Design review of the part built by this model. Coordinates are the model's own, in mm. A direction names the side the tool comes from. Coordinates: 2 decimals unless noted, no trailing zeros. Loops run counter-clockwise (first coordinate to the right, second up) from the corner with the lowest first, then second, coordinate; pieces in that order, holes last. Notation, with made-up numbers: (0, -20.5) - (51, -20.5) arc R11 cw to (51, -0.5) - close; hole circle Ø9 at (66, -3.75). An arc over 180 degrees is marked (long way). Answer in a Markdown table with one row per item. Add a question column.
(1) We need section C-C, the plane z = 31.5. Write out the cut boundary in (x, y), plus the area to 3 significant figures.
(2) Clearance check with flat-ended pins moving along their axes: pin 1 (4.5 mm diameter, centred on x = 10.5, y = -0.5, fed in from -Z); pin 2 (0.5 mm diameter, centred on x = -15.5, y = -4, fed in from -Z); pin 3 (12 mm diameter, centred on y = -0.5, z = 97, fed in from +X); pin 4 (1 mm diameter, centred on y = -4, z = 122, fed in from -X). State where each tip first meets the part, or that it passes through.
(3) To check wall thickness, follow L1, parallel to Z at x = 9, y = 8; L2, parallel to X at y = 0.5, z = 114; L3, parallel to Y at x = -0.5, z = 101. State the ranges of each line that lie inside material, in increasing order. Write a range as [from, to].
(4) For faces 1 (the face through (0, 14, 123)), 2 (the face through (-4.26, 0.03, 4.18)), 3 (the face through (-13.5, 0, 58)), 4 (the face through (11, 0, 8.477)), list the 3-axis set-ups (+Z, -Z, +X, -X, +Y, -Y) from which the entire face can be reached by the end or side of a thin tool; tool diameter is ignored.
(5) We need section B-B, the plane y = 5. Write out the cut boundary in (x, z), plus the area to 3 significant figures.
(6) The part is to be moulded in two halves that separate along X. For faces 5 (the face through (0, 2, 53)), 6 (the face through (0, -1, 108.5)), 7 (the face through (10.24, 0.03, 4.18)), say which applies: released by +X, released by -X, zero draft, split by the parting line, or undercut.
(7) We need section A-A, the plane x = 0.5. Write out the cut boundary in (y, z).
from build123d import *

# Parameters (mm, degrees)
ESQUISSE1_W             = 27
ESQUISSE1_H             = 4
BOSS_EXTRU_1_DEPTH      = 108
ENL_V_MAT_EXTRU_3_DEPTH = 109.913956865
ESQUISSE2_W             = 32
ESQUISSE2_H             = 30
BOSS_EXTRU_2_DEPTH      = 29
ESQUISSE17_W            = 27
ESQUISSE17_H            = 28
ENL_V_MAT_EXTRU_4_DEPTH = 29
ESQUISSE18_W            = 7
ESQUISSE18_H            = 2
ENL_V_MAT_EXTRU_6_DEPTH = 1
ESQUISSE24_W            = 7
ESQUISSE24_H            = 2
ENL_V_MAT_EXTRU_7_DEPTH = 1
ESQUISSE26_W            = 14
ESQUISSE26_H            = 7
ENL_V_MAT_EXTRU_8_DEPTH = 141.946798474


with BuildPart() as part:
    # Esquisse1 → Boss.-Extru.1 (new body)
    with BuildSketch(Plane.XY):
        Rectangle(ESQUISSE1_W, ESQUISSE1_H)
    extrude(amount=BOSS_EXTRU_1_DEPTH)

    # Esquisse12 → Enlèv. mat.-Extru.3 (cut, through all)
    with BuildSketch(Plane(origin=(0, 2, 0), x_dir=(1, 0, 0), z_dir=(0, 1, 0))):
        Polygon((-13.5, 0), (-11.207074173, 0), (-9.25, -8.477019564), (-13.5, -8.477019564), align=None)
        Polygon((-3.292925827, 0), (-5.25, -8.477019564), (5.25, -8.477019564), (3.292925827, 0), align=None)
        Polygon((11.207074173, 0), (9.25, -8.477019564), (13.5, -8.477019564), (13.5, 0), align=None)
    extrude(amount=-ENL_V_MAT_EXTRU_3_DEPTH, mode=Mode.SUBTRACT)

    # Esquisse2 → Boss.-Extru.2 (add)
    with BuildSketch(Plane.XY.offset(108)):
        Rectangle(ESQUISSE2_W, ESQUISSE2_H)
    extrude(amount=BOSS_EXTRU_2_DEPTH)

    # Esquisse17 → Enlèv. mat.-Extru.4 (cut)
    with BuildSketch(Plane.XZ.offset(15)):
        with Locations((0, 122.5)):
            Rectangle(ESQUISSE17_W, ESQUISSE17_H)
    extrude(amount=-ENL_V_MAT_EXTRU_4_DEPTH, mode=Mode.SUBTRACT)

    # Esquisse18 → Enlèv. mat.-Extru.6 (cut)
    with BuildSketch(Plane(origin=(16, 0, 0), x_dir=(0, 0, -1), z_dir=(1, 0, 0))):
        with Locations((-122.5, -4)):
            Rectangle(ESQUISSE18_W, ESQUISSE18_H)
    extrude(amount=-ENL_V_MAT_EXTRU_6_DEPTH, mode=Mode.SUBTRACT)

    # Esquisse24 → Enlèv. mat.-Extru.7 (cut)
    with BuildSketch(Plane.ZY.offset(16)):
        with Locations((122.5, -4)):
            Rectangle(ESQUISSE24_W, ESQUISSE24_H)
    extrude(amount=-ENL_V_MAT_EXTRU_7_DEPTH, mode=Mode.SUBTRACT)

    # Esquisse26 → Enlèv. mat.-Extru.8 (cut, through all)
    with BuildSketch(Plane.XZ.offset(-14)):
        with Locations((0, 118.5)):
            Rectangle(ESQUISSE26_W, ESQUISSE26_H)
    extrude(amount=-ENL_V_MAT_EXTRU_8_DEPTH, mode=Mode.SUBTRACT)


solid = part.part
Responses:
| question | item | result |
|---|---|---|
| 1 | outline | (-13.5, -2) - (13.5, -2) - (13.5, 2) - (-13.5, 2) - close |
| 1 | area | 108 mm2 |
| 2 | pin 1 | stops at z = 0 |
| 2 | pin 2 | stops at z = 108 |
| 2 | pin 3 | stops at x = 13.5 |
| 2 | pin 4 | stops at x = -15 |
| 3 | L1 | z = [108, 108.5], [136.5, 137] |
| 3 | L2 | x = [-16, -13.5], [13.5, 16] |
| 3 | L3 | y = [-2, 2] |
| 4 | face 1 | -Y |
| 4 | face 2 | +Y, -Y |
| 4 | face 3 | -Z, -X, +Y, -Y |
| 4 | face 4 | +X, +Y, -Y |
| 5 | outline | (-16, 108) - (16, 108) - (16, 137) - (-16, 137) - close; hole (-13.5, 108.5) - (13.5, 108.5) - (13.5, 136.5) - (-13.5, 136.5) - close |
| 5 | area | 172 mm2 |
| 6 | face 5 | zero draft |
| 6 | face 6 | undercut |
| 6 | face 7 | released by +X |
| 7 | outline | (-15, 108) - (-2, 108) - (-2, 8.48) - (2, 8.48) - (2, 108) - (15, 108) - (15, 115) - (14, 115) - (14, 108.5) - (-15, 108.5) - close; (-15, 136.5) - (14, 136.5) - (14, 122) - (15, 122) - (15, 137) - (-15, 137) - close |
